Geometry: final body of the model. Coordinates: model frame, mm. A direction names the side the tool comes from. Round coordinates to 2 decimals unless told otherwise and drop trailing zeros. Write each loop counter-clockwise with the first axis right and the second up, starting at its lowest first coordinate (ties: lowest second). Pieces come first, ordered by that corner, then holes. Notation, with made-up numbers: M 8,70.25 L 56,70.25 A22 ccw 56,88.25 Z; hole C 1.25,55.25 d10. An arc over 180 degrees is marked long. Use one line per item in the form item = value. Start each with the question number.
Item 1: Pin query (flat end, axial travel): pin 1 Ø2.5 at (x, y) = (51, 23.5) entering from +Z; pin 2 Ø4 at (x, z) = (39, 3) entering from +Y. Return the tip coordinate at first contact, or that it passes through.
Item 2: Section query D-D (y = 27.5). Return loops of the section in (x, z).
Item 3: Ray query, probe 1 along Y at (x, z) = (40, 7); probe 2 along X at (y, z) = (23.25, 4.5); probe 3 along Y at (x, z) = (23, 9.25). Return the intervals inside material, ascending.
Item 4: Section query C-C (x = 38). Return loops of the section in (y, z), and give its area (3 significant figures).
Item 5: Reachability of faces 4 (the flat face through (39, 34.043, 9)), 5 (the flat face through (40, 21.993, 6)), 6 (the cylindrical face through (47.674, 22.859, 9.577)), 7 (the flat face through (39, 16.543, 7)), 8 (the flat face through (23, 21.293, 10)) from +Z, -Z, +X, -X, +Y, -Y: full face, straight path, thin tool, end or side. Return the list, or none.
Item 6: Section query A-A (z = 5). Return loops of the section in (x, y), and give its area (3 significant figures).
Item 7: Pull-direction query (X, two-part tool) for faces 1 (the flat face through (20.849, 21, 6)), 2 (the flat face through (56.849, 25, 7)), 3 (the flat face through (40, 29.593, 6)); classes: pulls with the +X half, pulls with the -X half, needs draft (parallel to the pull), parting line crosses it, or undercut.
Item 8: Section query B-B (y = 24.5). Return loops of the section in (x, z).
from build123d import *

# Parameters (mm, degrees)
SKETCH1_W           = 36
SKETCH1_H           = 17.5
BOSS_EXTRUDE1_DEPTH = 15
SKETCH2_R           = 1.75
CUT_EXTRUDE1_DEPTH  = 15
SKETCH3_R           = 4
CUT_EXTRUDE2_DEPTH  = 11


with BuildPart() as part:
    # Sketch1 → Boss-Extrude1 (new body)
    with BuildSketch(Plane.XY):
        with Locations((38.848522366, 25.293010486)):
            Rectangle(SKETCH1_W, SKETCH1_H)
    extrude(amount=BOSS_EXTRUDE1_DEPTH)

    # Sketch2 → Cut-Extrude1 (cut)
    with BuildSketch(Plane.XY.offset(15)):
        with Locations((50.848522366, 25.293010486)):
            Circle(SKETCH2_R)
        with Locations((24.848522366, 25.293010486)):
            Circle(SKETCH2_R)
    extrude(amount=-CUT_EXTRUDE1_DEPTH, mode=Mode.SUBTRACT)

    # Sketch3 → Cut-Extrude2 (cut)
    with BuildSketch(Plane.XY.offset(15)):
        with Locations((50.848522366, 25.293010486)):
            Circle(SKETCH3_R)
        with BuildLine():
            Line((24.848522366, 29.293010486), (20.848522366, 29.293010486))
            Line((20.848522366, 29.293010486), (20.848522366, 21.293010486))
            Line((20.848522366, 21.293010486), (24.848522366, 21.293010486))
            ThreePointArc((24.848522366, 21.293010486), (28.848522366, 25.293010486), (24.848522366, 29.293010486))
        make_face()
    extrude(amount=-CUT_EXTRUDE2_DEPTH, mode=Mode.SUBTRACT)

    # Sketch4 → Cut-Revolve1 (revolve, cut)
    with BuildSketch(Plane.ZY.offset(-37.848522366)):
        Polygon((0, 16.543010486), (0, 34.293010486), (8.25, 34.293010486), (8.25, 29.593010486), (6, 29.593010486), (6, 24.993010486), (8.25, 24.993010486), (8.25, 21.993010486), (6, 21.993010486), (6, 16.543010486), align=None)
    revolve(axis=Axis((37.848522366, 16.543010486, 0), (0, 1, 0)), mode=Mode.SUBTRACT)


solid = part.part
Working result:
q1.pin_1 = 4
q1.pin_2 = through
q2.outline = M 20.85,0 L 31.85,0 A6 cw 43.85,0 L 56.85,0 L 56.85,15 L 54.18,15 L 54.18,4 L 47.51,4 L 47.51,15 L 28.18,15 L 28.18,4 L 20.85,4 Z
q3.probe_1 = 16.54 to 21.99, 24.99 to 29.59
q3.probe_2 = 28.29 to 30.93, 44.76 to 47.41, 54.29 to 56.85
q3.probe_3 = 16.54 to 21.29, 29.29 to 34.04
q4.outline = M 16.54,6 L 21.99,6 L 21.99,8.25 L 24.99,8.25 L 24.99,6 L 29.59,6 L 29.59,8.25 L 34.04,8.25 L 34.04,15 L 16.54,15 Z
q4.area = 141 mm²
q5.face_4 = +Z, -Z, +X, -X, +Y
q5.face_5 = -Z
q5.face_6 = +Z
q5.face_7 = +Z, -Z, +X, -X, -Y
q5.face_8 = +Z, -X
q6.outline = M 20.85,16.54 L 34.53,16.54 L 34.53,21.99 L 31.29,21.99 L 31.29,24.99 L 34.53,24.99 L 34.53,29.59 L 31.29,29.59 L 31.29,34.04 L 20.85,34.04 L 20.85,29.29 L 24.85,29.29 A4 cw 24.85,21.29 L 20.85,21.29 Z; M 41.17,16.54 L 56.85,16.54 L 56.85,34.04 L 44.41,34.04 L 44.41,29.59 L 41.17,29.59 L 41.17,24.99 L 44.41,24.99 L 44.41,21.99 L 41.17,21.99 Z; hole C 50.85,25.29 d8
q6.area = 358 mm²
q7.face_1 = pulls with the -X half
q7.face_2 = pulls with the +X half
q7.face_3 = undercut
q8.outline = M 20.85,0 L 23.29,0 L 23.29,4 L 20.85,4 Z; M 26.41,0 L 29.6,0 A8.25 cw 46.1,0 L 49.29,0 L 49.29,4 L 46.93,4 L 46.93,15 L 28.77,15 L 28.77,4 L 26.41,4 Z; M 52.41,0 L 56.85,0 L 56.85,15 L 54.77,15 L 54.77,4 L 52.41,4 Z
